Can you work these out from the drawing? Everything is in mm from the part's minimum corner. Give positions to 0.01 mm unless a question says otherwise; leave off trailing zeros. Loops run counter-clockwise (first coordinate to the right, second up) from the corner with the lowest first, then second, coordinate; pieces in that order, holes last.
Q1. If we section it at B-B (x = 18): Please give me the cut outline in (y, z), plus the area to 3 significant figures.
Q2. I need wall thicknesses on line 1 (X direction, y = 52, z = 1.6) (1 decimal); line 2 (X direction, y = 7, z = 2.9) (1 decimal). Which ranges of each line are inside material? Lowest first, please.
Q3. Will these pins go through, and if not, where does the flat tip stop? P1, Ø1.5, axis at y = 12.5, z = 0.5, coming from the -X side (1 decimal); P2, Ø2, axis at x = 30.5, z = 2, coming from the +Y side; P3, Ø2.5, axis at x = 95.5, z = 2, coming from the +Y side; P4, Ø2.5, axis at x = 50.97, y = 35.97, coming from the +Z side.
Q4. If we section it at A-A (z = 3.95): Give the number of separate pieces and of enclosed holes in the cut face, plus the area to 3 significant figures.
Q5. If we section it at C-C (y = 40): Please give me the cut outline in (x, z).
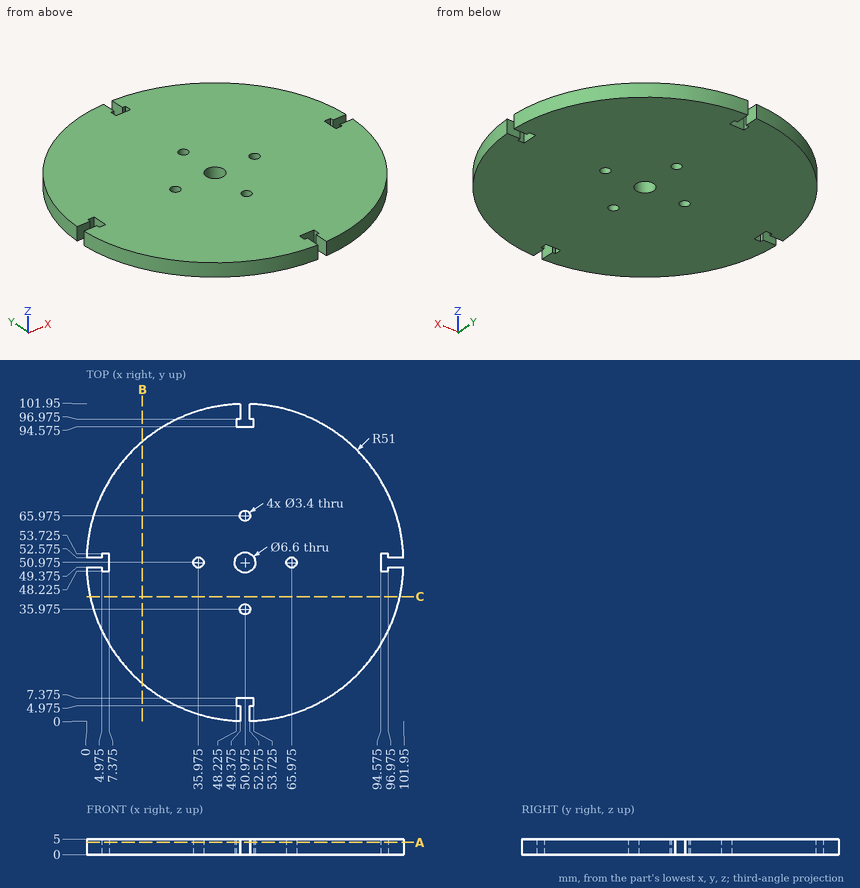
Check sheet entries:
1. outline: (12.07, 0) - (89.88, 0) - (89.88, 5) - (12.07, 5) - close
1. area: 389 mm2
2. line 1: x = 7.4 to 34.6, 37.3 to 47.8, 54.1 to 64.6, 67.3 to 94.6
2. line 2: x = 25.1 to 48.2, 53.7 to 76.8
3. P1: stops at x = 16.7
3. P2: stops at y = 98.11
3. P3: stops at y = 77.96
3. P4: passes through
4. separate pieces: 1
4. enclosed holes: 5
4. area: 7,980 mm2
5. outline: (1.17, 0) - (100.78, 0) - (100.78, 5) - (1.17, 5) - close
